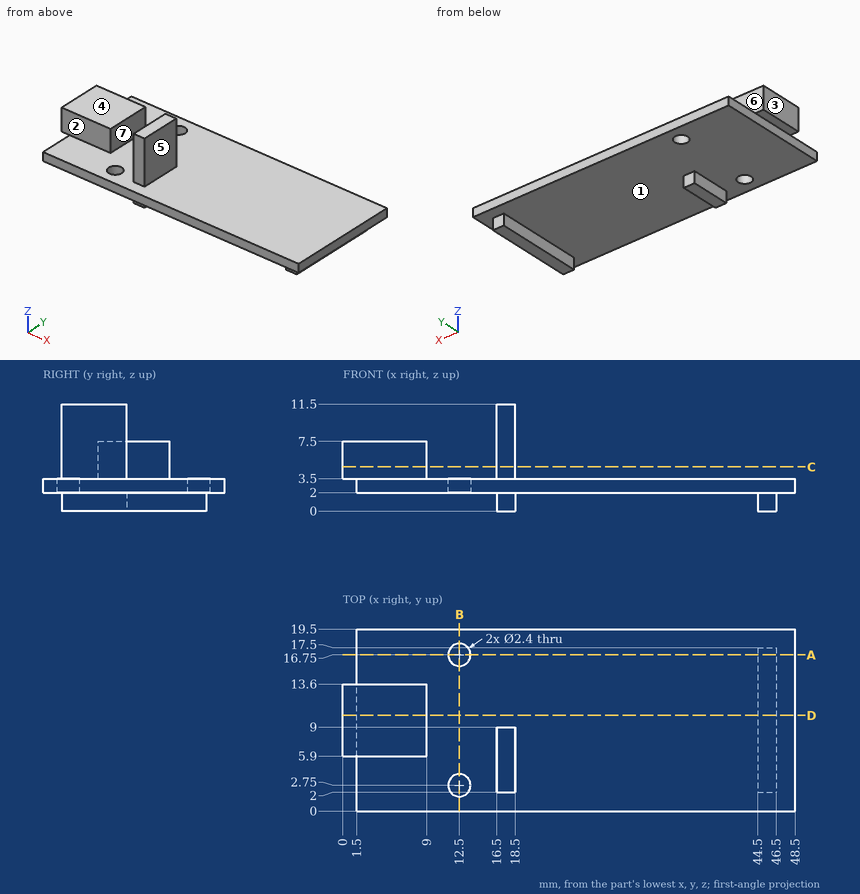
Could you check a few things on this drawing? It's one solid part, dimensions in mm from its lowest x, y, z. A direction names the side the tool comes from. Coordinates: 2 decimals unless noted, no trailing zeros. Order: outer loops, then holes, each group sorted by start corner. A loop starts at its lowest first (then second) coordinate and runs counter-clockwise, first axis right, second up. Notation, with made-up numbers: (58, -28) - (115, -28) arc R28 cw to (115, 1) - close; hole circle Ø8 at (50, 51). An arc over 180 degrees is marked (long way). Answer as a JSON object with one key per item and string values. Group by question number.
Q1. I need wall thicknesses on line 1 (Y direction, x = 12.5, z = 3.1); line 2 (X direction, y = 4.5, z = 1.5); line 3 (Z direction, x = 28.5, y = 17.25). Which ranges of each line are inside material? Lowest first, please. Write a range as from..to.
Q2. Imagine slicing it at B-B (x = 12.5). Please give me the cut outline in (y, z).
Q3. Imagine slicing it at A-A (y = 16.75). Please give me the cut outline in (x, z).
Q4. We'd pull the mould along X, two halves only. Please class the marked faces 1, 2 and 3: +X half, -X half, draft (parallel to the pull), parting line (faces both ways), or undercut.
Q5. On a 3-axis mill with a long thin cutter (end or side, diameter ignored), from which of +Z, -Z, +X, -X, +Y, -Y can I reach the whole of each face in a straight line? I mean the marked faces 4, 5, 6 and 7. Say none if no direction works.
Q6. Will these pins go through, and if not, where does the flat tip stop? P1, Ø1.6, axis at x = 0.5, y = 9.5, coming from the -Z side; P2, Ø0.6, axis at y = 8.5, z = 1, coming from the -X side; P3, Ø1.5, axis at y = 11, z = 7.5, coming from the +X side.
Q7. Imagine slicing it at D-D (y = 10.25). Please give me the cut outline in (x, z).
Q8. Imagine slicing it at C-C (z = 4.75). Please give me the cut outline in (x, y), and give its area (3 significant figures).
Determined:
{
 "1": {"line 1": "y = 0..1.55, 3.95..15.55, 17.95..19.5", "line 2": "x = 16.5..18.5, 44.5..46.5", "line 3": "z = 2..3.5"},
 "2": {"outline": "(0, 2) - (1.55, 2) - (1.55, 3.5) - (0, 3.5) - close; (3.95, 2) - (15.55, 2) - (15.55, 3.5) - (3.95, 3.5) - close; (17.95, 2) - (19.5, 2) - (19.5, 3.5) - (17.95, 3.5) - close"},
 "3": {"outline": "(1.5, 2) - (11.3, 2) - (11.3, 3.5) - (1.5, 3.5) - close; (13.7, 2) - (44.5, 2) - (44.5, 0) - (46.5, 0) - (46.5, 2) - (48.5, 2) - (48.5, 3.5) - (13.7, 3.5) - close"},
 "4": {"face 1": "undercut", "face 2": "draft", "face 3": "-X half"},
 "5": {"face 4": "+Z, -X, +Y, -Y", "face 5": "+Z, +X, +Y, -Y", "face 6": "+Z, +X, -X, +Y", "face 7": "+Z, +Y, -Y"},
 "6": {"P1": "stops at z = 3.5", "P2": "stops at x = 16.5", "P3": "stops at x = 9"},
 "7": {"outline": "(0, 3.5) - (1.5, 3.5) - (1.5, 2) - (44.5, 2) - (44.5, 0) - (46.5, 0) - (46.5, 2) - (48.5, 2) - (48.5, 3.5) - (9, 3.5) - (9, 7.5) - (0, 7.5) - close"},
 "8": {"outline": "(0, 5.9) - (9, 5.9) - (9, 13.6) - (0, 13.6) - close; (16.5, 2) - (18.5, 2) - (18.5, 9) - (16.5, 9) - close", "area": "83.3 mm2"}
}
